Here's how the part is built. I have some questions about the finished solid (model axes, mm). A direction names the side the tool comes from. Give positions to 0.01 mm unless a question says otherwise; leave off trailing zeros. Write each loop counter-clockwise with the first axis right and the second up, starting at its lowest first coordinate (ties: lowest second). Pieces come first, ordered by that corner, then holes. Notation, with made-up numbers: (-21, -38.75) -> (-6, -38.75) arc R26 cw to (-6, -22.75) -> close; hole circle Ø10 at (-16.75, -24). An arc over 180 degrees is marked (long way). Return JSON: item names as keys, results as strings.
from build123d import *

# Parameters (mm, degrees)
SKETCH1_W           = 40
SKETCH1_H           = 40
BOSS_EXTRUDE1_DEPTH = 15
SKETCH3_R           = 2.75
BOSS_EXTRUDE2_DEPTH = 5
FILLET1_R           = 1
SKETCH4_R           = 12.5
CUT_EXTRUDE1_DEPTH  = 3.5
SKETCH5_R           = 5
CUT_EXTRUDE2_DEPTH  = 41
SKETCH6_R           = 3
CUT_EXTRUDE3_DEPTH  = 2
SKETCH7_R           = 1.75
CUT_EXTRUDE4_DEPTH  = 16


with BuildPart() as part:
    # Sketch1 → Boss-Extrude1 (new body)
    with BuildSketch(Plane.XY):
        Rectangle(SKETCH1_W, SKETCH1_H)
    extrude(amount=BOSS_EXTRUDE1_DEPTH)

    # Sketch3 → Boss-Extrude2 (add)
    with BuildSketch(Plane(origin=(0, 0, 0), x_dir=(-1, 0, 0), z_dir=(0, 0, -1))):
        with Locations(Location((-15, 15, 0), (0, 0, 180))):  # turned: the seam where the file's is
            Circle(SKETCH3_R)
        with Locations(Location((15, 15, 0), (0, 0, 180))):  # turned: the seam where the file's is
            Circle(SKETCH3_R)
        with Locations(Location((-15, -15, 0), (0, 0, 180))):  # turned: the seam where the file's is
            Circle(SKETCH3_R)
        with Locations(Location((15, -15, 0), (0, 0, 180))):  # turned: the seam where the file's is
            Circle(SKETCH3_R)
    extrude(amount=BOSS_EXTRUDE2_DEPTH)

    # Fillet1
    fillet1_edges = [part.edges().sort_by_distance(p)[0] for p in [
        (12.25, 15, -5),
        (-17.75, 15, -5),
        (12.25, -15, -5),
        (-17.75, -15, -5),
    ]]
    fillet(fillet1_edges, radius=FILLET1_R)

    # Sketch4 → Cut-Extrude1 (cut)
    with BuildSketch(Plane(origin=(0, 0, 0), x_dir=(-1, 0, 0), z_dir=(0, 0, -1))):
        Circle(SKETCH4_R)
    extrude(amount=-CUT_EXTRUDE1_DEPTH, mode=Mode.SUBTRACT)

    # Sketch5 → Cut-Extrude2 (cut, through all)
    with BuildSketch(Plane(origin=(0, 20, 0), x_dir=(1, 0, 0), z_dir=(0, 1, 0))):
        with Locations((0, -16.5)):
            Circle(SKETCH5_R)
    extrude(amount=-CUT_EXTRUDE2_DEPTH, mode=Mode.SUBTRACT)

    # Sketch6 → Cut-Extrude3 (cut)
    with BuildSketch(Plane(origin=(0, 0, 0), x_dir=(-1, 0, 0), z_dir=(0, 0, -1))):
        with Locations((-16.5, 0)):
            Circle(SKETCH6_R)
        with Locations((16.5, 0)):
            Circle(SKETCH6_R)
    extrude(amount=-CUT_EXTRUDE3_DEPTH, mode=Mode.SUBTRACT)

    # Sketch7 → Cut-Extrude4 (cut, through all)
    with BuildSketch(Plane(origin=(0, 0, 0), x_dir=(-1, 0, 0), z_dir=(0, 0, -1))):
        with Locations((16.5, 0)):
            Circle(SKETCH7_R)
        with Locations((-16.5, 0)):
            Circle(SKETCH7_R)
    extrude(amount=-CUT_EXTRUDE4_DEPTH, mode=Mode.SUBTRACT)


solid = part.part
1. Suppose I cut it at D-D, the plane y = 15. List the corners of the cut face in (x, z) for me, and give its area (3 significant figures).
Taken from the geometry:
{"outline": "(-20, 0) -> (-17.75, 0) -> (-17.75, -4) arc R1 ccw to (-16.75, -5) -> (-13.25, -5) arc R1 ccw to (-12.25, -4) -> (-12.25, 0) -> (12.25, 0) -> (12.25, -4) arc R1 ccw to (13.25, -5) -> (16.75, -5) arc R1 ccw to (17.75, -4) -> (17.75, 0) -> (20, 0) -> (20, 15) -> (4.77, 15) arc R5 cw to (-4.77, 15) -> (-20, 15) -> close", "area": "630 mm²"}
2. Suppose I cut it at A-A, the plane y = 3.5. List the corners of the cut face in (x, z) for me, and give its area (3 significant figures).
Taken from the geometry:
{"outline": "(-20, 0) -> (-12, 0) -> (-12, 3.5) -> (12, 3.5) -> (12, 0) -> (20, 0) -> (20, 15) -> (4.77, 15) arc R5 cw to (-4.77, 15) -> (-20, 15) -> close", "area": "492 mm²"}
3. For pin 1 Ø5 at (x, y) = (-5.5, -1) entering from -Z; pin 2 Ø4 at (x, y) = (-16.5, 0) entering from -Z; pin 3 Ø6.5 at (x, y) = (-15.5, -1) entering from -Z, each with a flat end and sliding along its axis, tell me the tip position at first contact or that it passes through.
Taken from the geometry:
{"pin 1": "stops at z = 3.5", "pin 2": "stops at z = 2", "pin 3": "stops at z = 0"}
4. Which directions (+Z, -Z, +X, -X, +Y, -Y) give clear straight access to the entire face, cutting with the end or side of a thin tool? Please do faces 4 (the face through (12, 0, 15)), 5 (the face through (19.5, 0.1, 1)).
Taken from the geometry:
{"face 4": "+Z, +X, -X, +Y, -Y", "face 5": "-Z"}
5. If I drill on line 1 (Y direction, x = 0, z = 1.4); line 2 (X direction, y = 1, z = 10.75); line 3 (Z direction, x = -16, y = 11), over which ranges is the centre line in solid material (lowest first)? Write a range as [from, to].
Taken from the geometry:
{"line 1": "y = [-20, -12.5], [12.5, 20]", "line 2": "x = [-20, -17.94], [-15.06, 15.06], [17.94, 20]", "line 3": "z = [0, 15]"}
6. If we mould it in two halves opening along Y, with no side actions, what happens to faces 1 (the face through (0, 20, 7)), 2 (the face through (15, 15, -5)), 3 (the face through (12.973, 13.141, -1.972))? For each: released by +Y, released by -Y, zero draft, split by the parting line, or undercut.
Taken from the geometry:
{"face 1": "released by +Y", "face 2": "zero draft", "face 3": "undercut"}
7. Suppose I cut it at B-B, the plane x = 0. List the corners of the cut face in (y, z) for me.
Taken from the geometry:
{"outline": "(-20, 0) -> (-12.5, 0) -> (-12.5, 3.5) -> (12.5, 3.5) -> (12.5, 0) -> (20, 0) -> (20, 11.5) -> (-20, 11.5) -> close"}
8. Suppose I cut it at C-C, the plane z = -2.75. List the corners of the cut face in (x, y) for me, and give its area (3 significant figures).
Taken from the geometry:
{"outline": "circle Ø5.5 at (-15, -15); circle Ø5.5 at (-15, 15); circle Ø5.5 at (15, -15); circle Ø5.5 at (15, 15)", "area": "95.0 mm²"}
